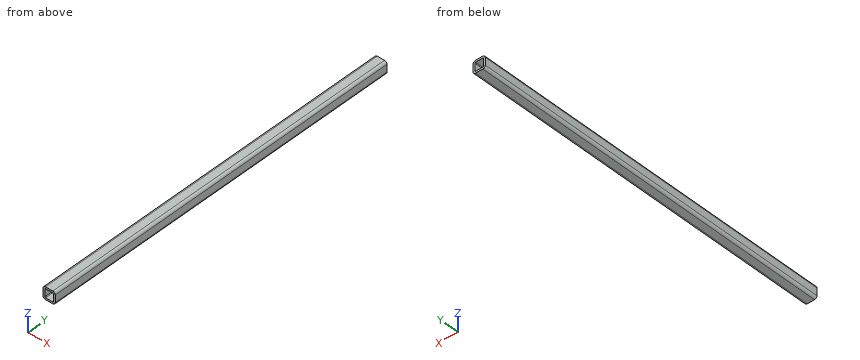
```python
from build123d import *

# Parameters (mm, degrees)
F0_W     = 10
F0_H     = 10
F1_DEPTH = 300
F2_R     = 2
F3_T     = -1.5


with BuildPart() as f1:
    # F0 (on Front) → F1 (new body)
    with BuildSketch(Plane.XZ):
        with Locations((65.800157, 14.793174)):
            Rectangle(F0_W, F0_H)
    extrude(amount=F1_DEPTH)

    # F2
    f2_edges = [f1.edges().sort_by_distance(p)[0] for p in [
        (70.800157, -150, 19.793174),
        (60.800157, -150, 19.793174),
        (70.800157, -150, 9.793174),
        (60.800157, -150, 9.793174),
    ]]
    fillet(f2_edges, radius=F2_R)

    # F3
    f3_openings = [f1.faces().sort_by_distance(p)[0] for p in [
        (65.800157, -300, 14.793174),
        (65.800157, 0, 14.793174),
    ]]
    offset(amount=F3_T, openings=f3_openings)


solid = f1.part
```
Input: part model. Units: mm. Frame: model coordinates. Round coordinates to 2 decimals unless told otherwise and drop trailing zeros. Loops run counter-clockwise (first coordinate to the right, second up) from the corner with the lowest first, then second, coordinate; pieces in that order, holes last. Notation, with made-up numbers: (30.25, 85.5) - (57.25, 85.5) arc R20 cw to (57.25, 104.5) - close; hole circle Ø2 at (8.25, 81). An arc over 180 degrees is marked (long way). One line per item, written item: value. Start each with the question number.
(1) Ray query, line 1 (Z direction, x = 68.25, y = -240); line 2 (X direction, y = -96.5, z = 15.5); line 3 (X direction, y = -120, z = 11.5). Return the intervals inside material, ascending. Write a range as [from, to].
(2) Section B-B, the plane y = -41.5. Return loops of the section in (x, z), plus the area to 3 significant figures.
(3) Section A-A, the plane z = 14. Return loops of the section in (x, y).
Results below:
1. line 1: [9.79, 11.29], [18.29, 19.79]
1. line 2: [60.8, 62.3], [69.3, 70.8]
1. line 3: [60.82, 62.4], [69.21, 70.78]
2. outline: (60.8, 11.79) arc R2 ccw to (62.8, 9.79) - (68.8, 9.79) arc R2 ccw to (70.8, 11.79) - (70.8, 17.79) arc R2 ccw to (68.8, 19.79) - (62.8, 19.79) arc R2 ccw to (60.8, 17.79) - close; hole (62.3, 11.79) arc R0.5 ccw to (62.8, 11.29) - (68.8, 11.29) arc R0.5 ccw to (69.3, 11.79) - (69.3, 17.79) arc R0.5 ccw to (68.8, 18.29) - (62.8, 18.29) arc R0.5 ccw to (62.3, 17.79) - close
2. area: 47.8 mm^2
3. outline: (60.8, -300) - (62.3, -300) - (62.3, 0) - (60.8, 0) - close; (69.3, -300) - (70.8, -300) - (70.8, 0) - (69.3, 0) - close
